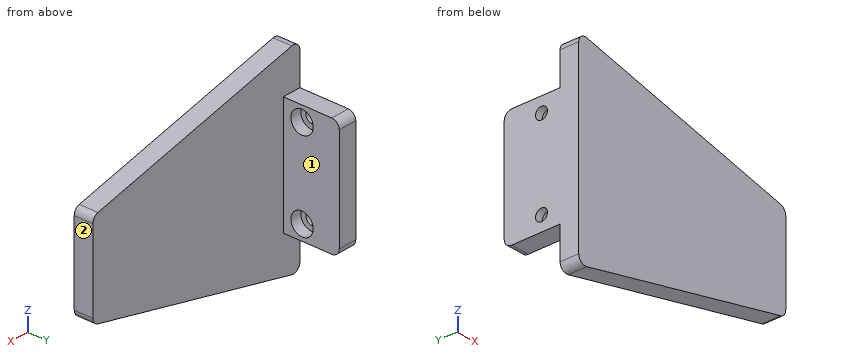
Autodesk Inventor part; units mm, degrees
ref_plane "YZ Plane" through (0, 0, 0) normal (1, 0, 0) x (0, 1, 0)
ref_plane "XZ Plane" through (0, 0, 0) normal (0, 1, 0) x (-1, 0, 0)
ref_plane "XY Plane" through (0, 0, 0) normal (0, 0, 1) x (1, 0, 0)
sketch "スケッチ1" plane through (0, 0, 0) normal (0, 1, 0) x (-1, 0, 0)
  line L0 (0, 0) -> (0, 54)
  line L1 (0, 54) -> (-62.76, 39.5107)
  line L2 (-62.76, 39.5107) -> (-62.76, 14.4893)
  line L3 (-62.76, 14.4893) -> (0, 0)
  dimension "d0" = 77
  dimension "d1" = 77
  dimension "d2" = 62.76
  dimension "d3" = 54
extrude "押し出し1" add sketch "スケッチ1" along normal blind 5
sketch "スケッチ2" plane through (0, 0, 0) normal (-1, 0, 0) x (0, 0, 1)
  line L0 (39.5107, 5) -> (14.4893, 5)
  line L1 (42.75, 5) -> (11.25, 5)
  line L2 (11.25, 5) -> (11.25, 20)
  line L3 (11.25, 20) -> (42.75, 20)
  line L4 (42.75, 20) -> (42.75, 5)
  line L5 (54, 0) -> (54, 5)
  point P0 (0, 0)
  dimension "d6" = 31.5
  dimension "d7" = 15
  dimension "d8" = 11.25
extrude "押し出し2" add sketch "スケッチ2" against normal blind 5
sketch "スケッチ3" plane through (5, 0, 0) normal (1, 0, 0) x (0, 0, -1)
  line L0 (-42.75, 20) -> (-42.75, 5)
  line L1 (-39.5107, 5) -> (-14.4893, 5)
  point P0 (0, 0)
  point P1 (-38.75, 10)
  point P2 (-15.25, 10)
  dimension "d15" = 10
  dimension "d11" = 4
  dimension "d12" = 5
  dimension "d18" = 23.5
hole "穴1" at (5, 10, 38.75) at (5, 10, 15.25) direction (-1, 0, 0) diameter 3.2 depth 8 tip angle 118 counterbore diameter 6 counterbore depth 3
fillet "フィレット1" radius 2 6 edges at (0, 2.5, 54) (0, 2.5, 0) (62.76, 2.5, 14.4893) (62.76, 2.5, 39.5107) (2.5, 20, 42.75) (2.5, 20, 11.25)
equation "\"d1\" = d0"
properties part number "nail" material "ABS プラスチック"
Design review of the part built by this model. Coordinates are the model's own, in mm. Face numbers are marked on the shaded views. A direction names the side the tool comes from. Coordinates: 2 decimals unless noted, no trailing zeros. Order: outer loops, then holes, each group sorted by start corner. A loop starts at its lowest first (then second) coordinate and runs counter-clockwise, first axis right, second up. Notation, with made-up numbers: (-20.5, 29) - (7.5, 29) arc R13 ccw to (7.5, 41) - close; hole circle Ø1 at (48.25, 24). An arc over 180 degrees is marked (long way). Put each result on its own line as item: value.
1) Insertion check: P1, Ø10, axis at x = 8, y = 14.5, coming from the +Z side; P2, Ø1.5, axis at x = 21, z = 21.5, coming from the -Y side; P3, Ø3.5, axis at y = 10, z = 38.75, coming from the +X side; P4, Ø5.5, axis at x = 3.5, y = 10.5, coming from the -Z side. Each pin has a flat end and moves straight along its axis. Give the tip position at first contact, or say it passes through.
Response values:
P1: stops at z = 42.75
P2: stops at y = 0
P3: stops at x = 2
P4: stops at z = 11.25
2) Wall thickness on L1, parallel to Z at x = 3.45, y = 10; L2, parallel to Z at x = 1.35, y = 10; L3, parallel to Y at x = 1.65, z = 38.75: over which ranges is each line inside the solid? List them lowest first. Write a range as from..to.
Response values:
L1: z = 11.25..12.25, 18.25..35.75, 41.75..42.75
L2: z = 11.25..13.65, 16.85..37.15, 40.35..42.75
L3: y = 0..8.4, 11.6..20
3) Tool access review of the marked faces 1 and 2: name each direction out of +Z, -Z, +X, -X, +Y, -Y from which nothing blocks a thin tool from reaching the whole face with its end or side.
Response values:
face 1: +Z, -Z, +X, +Y
face 2: +Z, -Z, +X, +Y, -Y
4) Take a section at D-D, the plane x = 18. Give the boundary of the cut face in (y, z), and give its area (3 significant figures).
Response values:
outline: (0, 4.16) - (5, 4.16) - (5, 49.84) - (0, 49.84) - close
area: 228 mm²
5) Take a section at B-B, the plane z = 32. Give the boundary of the cut face in (x, y).
Response values:
outline: (0, 0) - (62.76, 0) - (62.76, 5) - (5, 5) - (5, 20) - (0, 20) - close
6) Take a section at C-C, the plane z = 38.75. Give the boundary of the cut face in (x, y), and give its area (3 significant figures).
Response values:
outline: (0, 0) - (62.58, 0) - (62.58, 5) - (5, 5) - (5, 7) - (2, 7) - (2, 8.4) - (0, 8.4) - close; (0, 11.6) - (2, 11.6) - (2, 13) - (5, 13) - (5, 20) - (0, 20) - close
area: 363 mm²
7) Take a section at A-A, the plane y = 10. Give the boundary of the cut face in (x, z).
Response values:
outline: (0, 11.25) - (5, 11.25) - (5, 12.25) - (2, 12.25) - (2, 13.65) - (0, 13.65) - close; (0, 16.85) - (2, 16.85) - (2, 18.25) - (5, 18.25) - (5, 35.75) - (2, 35.75) - (2, 37.15) - (0, 37.15) - close; (0, 40.35) - (2, 40.35) - (2, 41.75) - (5, 41.75) - (5, 42.75) - (0, 42.75) - close
